CAD build for the part. Positions are in the model's coordinates, mm. Face numbers are marked on the shaded views. A direction names the side the tool comes from. Give positions to 0.01 mm unless a question says otherwise; leave off trailing zeros. Loops run counter-clockwise (first coordinate to the right, second up) from the corner with the lowest first, then second, coordinate; pieces in that order, holes last. Notation, with made-up numbers: M 0,-9 L 4,-9 A15 cw 4,2 Z; hole C -30.5,59 d3. An arc over 180 degrees is marked long. Answer as CSV lines item,"result".
```python
from build123d import *

# Parameters (mm, degrees)
SKETCH2_W            = 38
SKETCH2_H            = 11.4
BOSS_EXTRUDE1_DEPTH  = 1.45
SKETCH1_R            = 3.0875
BOSS_EXTRUDE2_DEPTH  = 1.55
SKETCH4_W            = 11.1
SKETCH4_H            = 3.15
CUT_EXTRUDE1_DEPTH   = 1.55
SKETCH5_R            = 2.5
BOSS_EXTRUDE3_DEPTH  = 0.5
SKETCH6_W            = 2.1
SKETCH6_H            = 6.8
BOSS_EXTRUDE4_DEPTH  = 5.5
BOSS_EXTRUDE5_DEPTH  = 2.1
SKETCH10_W           = 1.8
SKETCH10_H           = 1.137503558
CUT_EXTRUDE2_DEPTH   = 13.5
BOSS_EXTRUDE6_START  = -3.325
BOSS_EXTRUDE6_DEPTH  = 6.65
SKETCH13_W           = 1.609894421
SKETCH13_H           = 2.787309827
SKETCH13_H_2         = 3.919277545
CUT_EXTRUDE3_DEPTH   = 4.25
SKETCH14_R           = 2.399672092
SKETCH14_R_2         = 1.55
BOSS_EXTRUDE9_DEPTH  = 1.75
SKETCH15_R           = 1.55
BOSS_EXTRUDE10_DEPTH = 13.2
SKETCH19_W           = 4.15
SKETCH19_H           = 0.9812524
BOSS_EXTRUDE11_DEPTH = 5.5
FILLET1_R            = 3
FILLET2_R            = 0.5
CHAMFER1_SIZE        = 1
SKETCH20_R           = 2.45
CUT_EXTRUDE4_DEPTH   = 3.125
SKETCH21_R           = 3.0875
CUT_EXTRUDE5_DEPTH   = 0.8
FILLET5_R            = 0.4


# Read off the part's stored shape, not the designer's step: Boss-Extrude6
with BuildPart() as part:
    # Sketch2 → Boss-Extrude1 (new body)
    with BuildSketch(Plane(origin=(0, 0, 0), x_dir=(1, 0, 0), z_dir=(0, 1, 0))):
        Rectangle(SKETCH2_W, SKETCH2_H)
    extrude(amount=-BOSS_EXTRUDE1_DEPTH)

    # Sketch1 → Boss-Extrude2 (add)
    # profile 1 of 3: a face of its own
    with BuildSketch(Plane(origin=(0, 0, 0), x_dir=(1, 0, 0), z_dir=(0, 1, 0))):
        with BuildLine():
            ThreePointArc((-2.449489743, 0.5), (-2.5, 0), (-2.449489743, -0.5))
            Line((-2.449489743, -0.5), (-4.525137715, -0.5))
            ThreePointArc((-4.525137715, -0.5), (-4.870238296, -1.60440726), (-5.55, -2.540747921))
            Line((-5.55, -2.540747921), (-5.55, -5.7))
            Line((-5.55, -5.7), (-7.1, -5.7))
            Line((-7.1, -5.7), (-7.1, -4.45))
            Line((-7.1, -4.45), (-19, -4.45))
            Line((-19, -4.45), (-19, -3.45))
            Line((-19, -3.45), (-9.002083241, -3.45))
            ThreePointArc((-9.002083241, -3.45), (-10.745743425, -2.365214512), (-11.604862285, -0.5))
            Line((-11.604862285, -0.5), (-19, -0.5))
            Line((-19, -0.5), (-19, 0.5))
            Line((-19, 0.5), (-11.604862285, 0.5))
            ThreePointArc((-11.604862285, 0.5), (-10.745743425, 2.365214512), (-9.002083241, 3.45))
            Line((-9.002083241, 3.45), (-19, 3.45))
            Line((-19, 3.45), (-19, 4.45))
            Line((-19, 4.45), (-6.875, 4.45))
            Line((-6.875, 4.45), (-6.875, 5.7))
            Line((-6.875, 5.7), (-4.975, 5.7))
            Line((-4.975, 5.7), (-4.975, 4.45))
            Line((-4.975, 4.45), (4.975, 4.45))
            Line((4.975, 4.45), (4.975, 5.7))
            Line((4.975, 5.7), (6.875, 5.7))
            Line((6.875, 5.7), (6.875, 4.45))
            Line((6.875, 4.45), (19, 4.45))
            Line((19, 4.45), (19, 3.45))
            Line((19, 3.45), (9.002083241, 3.45))
            ThreePointArc((9.002083241, 3.45), (10.745743425, 2.365214512), (11.604862285, 0.5))
            Line((11.604862285, 0.5), (19, 0.5))
            Line((19, 0.5), (19, -0.5))
            Line((19, -0.5), (11.604862285, -0.5))
            ThreePointArc((11.604862285, -0.5), (10.745743425, -2.365214512), (9.002083241, -3.45))
            Line((9.002083241, -3.45), (19, -3.45))
            Line((19, -3.45), (19, -4.45))
            Line((19, -4.45), (7.1, -4.45))
            Line((7.1, -4.45), (7.1, -5.7))
            Line((7.1, -5.7), (5.55, -5.7))
            Line((5.55, -5.7), (5.55, -2.540747921))
            ThreePointArc((5.55, -2.540747921), (4.870238296, -1.60440726), (4.525137715, -0.5))
            Line((4.525137715, -0.5), (2.449489743, -0.5))
            ThreePointArc((2.449489743, -0.5), (2.5, 0), (2.449489743, 0.5))
            Line((2.449489743, 0.5), (4.525137715, 0.5))
            ThreePointArc((4.525137715, 0.5), (5.384256575, 2.365214512), (7.127916759, 3.45))
            Line((7.127916759, 3.45), (-7.127916759, 3.45))
            ThreePointArc((-7.127916759, 3.45), (-5.384256575, 2.365214512), (-4.525137715, 0.5))
            Line((-4.525137715, 0.5), (-2.449489743, 0.5))
        make_face()
        with Locations((8.065, 0)):
            Circle(SKETCH1_R, mode=Mode.SUBTRACT)
        with Locations((-8.065, 0)):
            Circle(SKETCH1_R, mode=Mode.SUBTRACT)
    # profile 2 of 3: a face of its own
    with BuildSketch(Plane(origin=(0, 0, 0), x_dir=(1, 0, 0), z_dir=(0, 1, 0))):
        with Locations((-8.065, 0)):
            Circle(SKETCH1_R)
    # profile 3 of 3: a face of its own
    with BuildSketch(Plane(origin=(0, 0, 0), x_dir=(1, 0, 0), z_dir=(0, 1, 0))):
        with Locations((8.065, 0)):
            Circle(SKETCH1_R)
    extrude(amount=BOSS_EXTRUDE2_DEPTH)

    # Sketch4 → Cut-Extrude1 (cut)
    with BuildSketch(Plane(origin=(0, 0, 0), x_dir=(1, 0, 0), z_dir=(0, 1, 0))):
        with Locations((0, -4.125)):
            Rectangle(SKETCH4_W, SKETCH4_H)
    extrude(amount=-CUT_EXTRUDE1_DEPTH, mode=Mode.SUBTRACT)

    # Sketch5 → Boss-Extrude3 (add)
    with BuildSketch(Plane(origin=(0, 0, 0), x_dir=(1, 0, 0), z_dir=(0, 1, 0))):
        Circle(SKETCH5_R)
    extrude(amount=BOSS_EXTRUDE3_DEPTH)

    # Sketch6 → Boss-Extrude4 (add)
    with BuildSketch(Plane.XZ.offset(1.45)):
        with Locations((-4.375, -0.85)):
            Rectangle(SKETCH6_W, SKETCH6_H)
        with Locations((4.375, -0.85)):
            Rectangle(SKETCH6_W, SKETCH6_H)
    extrude(amount=BOSS_EXTRUDE4_DEPTH)

    # Sketch8 → Boss-Extrude5 (add)
    with BuildSketch(Plane(origin=(5.425, 0, 0), x_dir=(0, 0, -1), z_dir=(1, 0, 0))):
        with BuildLine():
            Line((3.824457799, 1.55), (3.169391593, -1.45))
            Line((3.169391593, -1.45), (4.25, -1.45))
            Line((4.25, -1.45), (4.25, -3.2))
            ThreePointArc((4.25, -3.2), (6.591222467, -2.434687171), (6.999675652, -4.863718328))
            ThreePointArc((6.999675652, -4.863718328), (6.917672859, -5.503870326), (7.462386809, -5.85))
            Line((7.462386809, -5.85), (8.635307609, -5.85))
            Line((8.635307609, -5.85), (8.99741287, -4.588093961))
            ThreePointArc((8.99741287, -4.588093961), (7.994798141, -1.171963485), (5.7, 1.55))
            Line((5.7, 1.55), (3.824457799, 1.55))
        make_face()
        with BuildLine():
            Line((4.25, -4.45), (4.25, -5.812496442))
            ThreePointArc((4.25, -5.812496442), (4.621012042, -5.404327986), (4.501999453, -4.865730337))
            ThreePointArc((4.501999453, -4.865730337), (4.360365271, -4.667342163), (4.25, -4.45))
        make_face()
    boss_extrude5 = extrude(amount=-BOSS_EXTRUDE5_DEPTH)

    # Sketch10 → Cut-Extrude2 (cut)
    with BuildSketch(Plane(origin=(5.425, 0, 0), x_dir=(0, 0, -1), z_dir=(1, 0, 0))):
        with Locations((3.35, -6.381248221)):
            Rectangle(SKETCH10_W, SKETCH10_H)
    extrude(amount=-CUT_EXTRUDE2_DEPTH, mode=Mode.SUBTRACT)

    # Mirror2: Boss-Extrude5 across plane
    add(boss_extrude5.mirror(Plane(origin=(0, 0, 0), x_dir=(0, 0, 1), z_dir=(1, 0, 0))))

    # Boss-Extrude6 outline → Boss-Extrude6 (add)
    with BuildSketch(Plane.YZ.offset(BOSS_EXTRUDE6_START)):
        with BuildLine():
            Line((0, -5.7), (-1.45, -5.7))
            Line((-1.45, -5.7), (-1.45, -8.137740985))
            ThreePointArc((-1.45, -8.137740985), (-0.702713526, -7.723414198), (0, -7.237309827))
            Line((0, -7.237309827), (0, -5.7))
        make_face()
    extrude(amount=BOSS_EXTRUDE6_DEPTH)

    # Sketch13 → Cut-Extrude3 (cut)
    with BuildSketch(Plane(origin=(0, 0, 0), x_dir=(1, 0, 0), z_dir=(0, 1, 0))):
        with Locations((-4.129947211, 5.843654913)):
            Rectangle(SKETCH13_W, SKETCH13_H)
        with Locations((4.129947211, 6.409638773)):
            Rectangle(SKETCH13_W, SKETCH13_H_2)
    extrude(amount=CUT_EXTRUDE3_DEPTH, mode=Mode.SUBTRACT)

    # Sketch14 → Boss-Extrude9 (add)
    # profile 1 of 3: a face of its own
    with BuildSketch(Plane(origin=(7.475, 0, 0), x_dir=(0, 0, -1), z_dir=(1, 0, 0))):
        with BuildLine():
            Line((-7.549815065, -6.320389595), (-2.55, -6.95))
            Line((-2.55, -6.95), (-1.989793561, -6.95))
            Line((-1.989793561, -6.95), (-1.989793561, -1.45))
            Line((-1.989793561, -1.45), (-2.55, -1.45))
            Line((-2.55, -1.45), (-5.7, -1.45))
            Line((-5.7, -1.45), (-7.383162468, -1.543546098))
            ThreePointArc((-7.383162468, -1.543546098), (-5.60092755, -2.196251792), (-4.850327908, -3.93952062))
            ThreePointArc((-4.850327908, -3.93952062), (-5.662711698, -5.739226706), (-7.549815065, -6.320389595))
        make_face()
    # profile 2 of 3: a face of its own
    with BuildSketch(Plane(origin=(7.475, 0, 0), x_dir=(0, 0, -1), z_dir=(1, 0, 0))):
        with Locations((-7.25, -3.93952062)):
            Circle(SKETCH14_R)
        with Locations((-7.25, -3.93952062)):
            Circle(SKETCH14_R_2, mode=Mode.SUBTRACT)
    # profile 3 of 3: a face of its own
    with BuildSketch(Plane(origin=(7.475, 0, 0), x_dir=(0, 0, -1), z_dir=(1, 0, 0))):
        with Locations((-7.25, -3.93952062)):
            Circle(SKETCH14_R_2)
    boss_extrude9 = extrude(amount=-BOSS_EXTRUDE9_DEPTH)

    # Mirror3: Boss-Extrude9 across plane
    add(boss_extrude9.mirror(Plane(origin=(0, 0, 0), x_dir=(0, 0, 1), z_dir=(1, 0, 0))))

    # Sketch15 → Boss-Extrude10 (add)
    with BuildSketch(Plane.ZY.offset(7.475)):
        with Locations((7.25, -3.93952062)):
            Circle(SKETCH15_R)
    extrude(amount=-BOSS_EXTRUDE10_DEPTH)

    # Sketch17 → Cut-Revolve4 (revolve, cut)
    with BuildSketch(Plane.XY):
        with BuildLine():
            Line((2.1, 0.5), (2.1, 0.710906592))
            Line((2.1, 0.710906592), (0, 1.053607594))
            Line((0, 1.053607594), (0, 0.183808769))
            ThreePointArc((0, 0.183808769), (1.061835309, 0.263299583), (2.1, 0.5))
        make_face()
    revolve(axis=Axis((0, 1.053607594, 0), (0, -1, 0)), mode=Mode.SUBTRACT)

    # Sketch19 → Boss-Extrude11 (add)
    with BuildSketch(Plane.XZ.offset(6.95)):
        with Locations((5.4, 2.0593738)):
            Rectangle(SKETCH19_W, SKETCH19_H)
    boss_extrude11 = extrude(amount=-BOSS_EXTRUDE11_DEPTH)

    # Mirror4: Boss-Extrude11 across plane
    add(boss_extrude11.mirror(Plane(origin=(0, 0, 0), x_dir=(0, 0, 1), z_dir=(1, 0, 0))))

    # Fillet1
    # the kernel refuses this fillet: 3 mm, written as the material it takes off along each edge
    with BuildSketch(Plane(origin=(7.475, -14.064026638, 1.5687476), x_dir=(-1, 0, 0), z_dir=(0, 1, 0))) as fillet1_piece_1:
        with BuildLine():
            CenterArc((3, 2.845610655), FILLET1_R, 180, 71.538541703)
            Line((0, 2.845610655), (0, 0))
            Line((0, 0), (2.05, 0))
        make_face()
    extrude(amount=12.614026638, mode=Mode.SUBTRACT)
    with BuildSketch(Plane(origin=(3.325, -1.45, 2.55), x_dir=(0, 0, -1), z_dir=(0, -1, 0))) as fillet1_piece_2:
        with BuildLine():
            CenterArc((2.939387691, 3), FILLET1_R, 191.536959033, 78.463040967)
            Line((0, 2.4), (0, 0))
            Line((0, 0), (2.939387691, 0))
        make_face()
    extrude(amount=12.848469228, mode=Mode.SUBTRACT)
    with BuildSketch(Plane(origin=(-3.325, -1.45, 2.55), x_dir=(0, 0, -1), z_dir=(0, -1, 0))) as fillet1_piece_3:
        with BuildLine():
            CenterArc((2.939387691, -3), FILLET1_R, 90, 78.463040967)
            Line((0, -2.4), (0, 0))
            Line((0, 0), (2.939387691, 0))
        make_face()
    extrude(amount=12.848469228, mode=Mode.SUBTRACT)
    with BuildSketch(Plane(origin=(-7.475, -14.064026638, 1.5687476), x_dir=(0, 0, 1), z_dir=(0, 1, 0))) as fillet1_piece_4:
        with BuildLine():
            CenterArc((2.845610655, 3), FILLET1_R, 198.461458297, 71.538541703)
            Line((0, 2.05), (0, 0))
            Line((0, 0), (2.845610655, 0))
        make_face()
    extrude(amount=12.614026638, mode=Mode.SUBTRACT)

    # Fillet2
    fillet2_edges = [part.edges().sort_by_distance(p)[0] for p in [
        (4.375, -4.588093961, -8.99741287),
        (4.375, -5.85, -8.635307609),
        (4.375, -6.95, -2.45),
        (-4.375, -6.95, -2.45),
        (-4.375, -5.85, -8.635307609),
        (-4.375, -4.588093961, -8.99741287),
    ]]
    fillet(fillet2_edges, radius=FILLET2_R)

    # Chamfer1
    chamfer1_edges = [part.edges().sort_by_distance(p)[0] for p in [
        (-2.5, 1.55, 0),
        (2.5, 1.55, 0),
        (-19, 1.55, -3.95),
        (-19, 1.55, 0),
        (-19, 1.55, 3.95),
        (19, 1.55, 3.95),
        (19, 1.55, 0),
        (19, 1.55, -3.95),
    ]]
    chamfer(chamfer1_edges, length=CHAMFER1_SIZE)

    # Sketch20 → Cut-Extrude4 (cut, symmetric)
    with BuildSketch(Plane(origin=(0, 0, 0), x_dir=(1, 0, 0), z_dir=(0, 1, 0))):
        with Locations(Location((-8.065, 0, 0), (0, 0, 270))):
            Circle(SKETCH20_R)
        with Locations(Location((8.065, 0, 0), (0, 0, 270))):
            Circle(SKETCH20_R)
    extrude(amount=CUT_EXTRUDE4_DEPTH, both=True, mode=Mode.SUBTRACT)

    # Sketch21 → Cut-Extrude5 (cut)
    with BuildSketch(Plane(origin=(0, 1.55, 0), x_dir=(1, 0, 0), z_dir=(0, 1, 0))):
        with Locations(Location((-8.065, 0, 0), (0, 0, 270))):
            Circle(SKETCH21_R)
        with Locations(Location((8.065, 0, 0), (0, 0, 270))):
            Circle(SKETCH21_R)
    extrude(amount=-CUT_EXTRUDE5_DEPTH, mode=Mode.SUBTRACT)

    # Fillet5
    fillet5_edges = [part.edges().sort_by_distance(p)[0] for p in [
        (5.425, -4.2, 1.5687476),
        (-5.425, -4.2, 1.5687476),
        (-5.725, -4.2, 2.55),
        (5.725, -4.2, 2.55),
    ]]
    fillet(fillet5_edges, radius=FILLET5_R)


solid = part.part
```
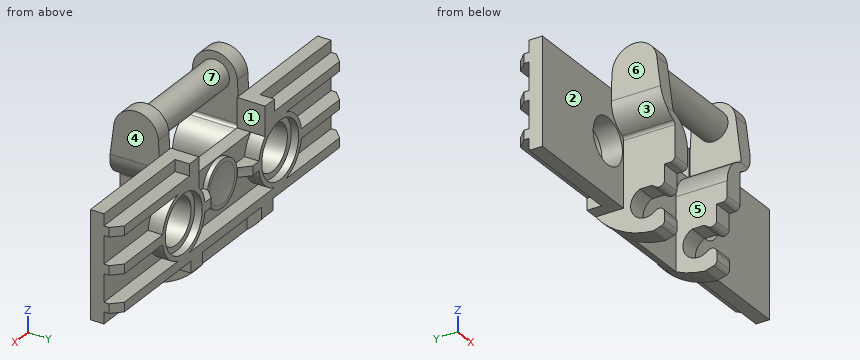
Q1. Cut at B-B (x = 14). Write the cut outline in (y, z), and give its area (3 significant figures).
Solution:
outline,"M -1.45,-5.7 L 0,-5.7 L 0,-4.45 L 1.55,-4.45 L 1.55,-3.45 L 0,-3.45 L 0,-0.5 L 1.55,-0.5 L 1.55,0.5 L 0,0.5 L 0,3.45 L 1.55,3.45 L 1.55,4.45 L 0,4.45 L 0,5.7 L -1.45,5.7 Z"
area,"21.2 mm²"
Q2. Cut at C-C (y = -0.5). Write the cut outline in (x, z) (3 decimals), and give its area (3 significant figures).
Solution:
outline,"M -19,-5.7 L -5.425,-5.7 L -5.425,-7.594 L 5.425,-7.594 L 5.425,-5.7 L 19,-5.7 L 19,5.7 L 5.55,5.7 L 5.55,2.55 L -5.55,2.55 L -5.55,5.7 L -19,5.7 Z; hole C -8.065,0 d4.9; hole C 8.065,0 d4.9"
area,"381 mm²"
Q3. Pin check, flat tips, straight feed: P1, Ø0.9, axis at x = -4, z = -3, coming from the -Y side; P2, Ø0.8, axis at x = 14.5, y = 1, coming from the -Z side; P3, Ø1.7, axis at y = -3.5, z = -3, coming from the +X side (3 decimals). Stop position of each tip, or through.
Solution:
P1,"stops at y = -5.81"
P2,"stops at z = -4.45"
P3,"stops at x = 5.425"
Q4. Cut at D-D (z = 0). Give the number of separate pieces and of enclosed holes in the cut face, and give its area (3 significant figures).
Solution:
separate pieces,"3"
enclosed holes,"0"
area,"97.2 mm²"
Q5. Which spindle directions (+Z, -Z, +X, -X, +Y, -Y) get a long thin tool onto all of the face, cutting with end or side? Do the marked faces 4, 5, 6 and 7. Say none if no direction does.
Solution:
face 4,"+Z, -Z, +X, -Y"
face 5,"-Z, -Y"
face 6,"+Z, -Z, -X, -Y"
face 7,"none"
Q6. Mould opens along X. For the marked faces 1, 2 and 3 say: released by +X, released by -X, zero draft, split by the parting line, or undercut.
Solution:
face 1,"undercut"
face 2,"zero draft"
face 3,"released by -X"
Q7. Wall check: line 1 (X direction, y = 0.1, z = 0) (3 decimals); line 2 (Z direction, x = 16, y = 0.5); line 3 (X direction, y = -4.5, z = 5.5) (3 decimals). Give the ranges that are in metal, low to high. Write a range as [from, to].
Solution:
line 1,"x = [-19, -10.515], [-5.615, 5.615], [10.515, 19]"
line 2,"z = [-4.45, -3.45], [-0.5, 0.5], [3.45, 4.45]"
line 3,"x = [-7.475, -5.725], [5.725, 7.475]"
Q8. Cut at A-A (x = 1). Write the cut outline in (y, z).
Solution:
outline,"C -3.94,7.25 d3.1; M -1.45,-8.14 A8.64 ccw 0,-7.24 L 0,-4.45 L 1.55,-4.45 L 1.55,-3.45 L 0,-3.45 L 0,-2.29 L 0.5,-2.29 L 0.5,-1.85 A7.06 cw 0.5,1.85 L 0.5,2.29 L 0,2.29 L 0,2.55 L -1.45,2.55 Z"
